from build123d import *

# Parameters (mm, degrees)
SKETCH_W      = 85
SKETCH_H      = 56
SKETCH_R      = 1.35
PAD_DEPTH     = 4
SKETCH001_W   = 50
SKETCH001_H   = 5
PAD001_DEPTH  = 8.5
SKETCH002_W   = 50
SKETCH002_H   = 5
SKETCH002_W_2 = 48
SKETCH002_H_2 = 3
POCKET_DEPTH  = 6
SKETCH003_W   = 17.5
SKETCH003_H   = 12
PAD002_DEPTH  = 16
SKETCH004_W   = 21.1
SKETCH004_H   = 16
PAD003_DEPTH  = 13.5
SKETCH005_W   = 9.2
SKETCH005_H   = 10.5
PAD004_DEPTH  = 3.2
SKETCH006_W   = 7
SKETCH006_H   = 8
PAD005_DEPTH  = 3
SKETCH007_W   = 7
SKETCH007_H   = 12
PAD006_DEPTH  = 6


with BuildPart() as part:
    # Sketch → Pad (new body)
    with BuildSketch(Plane.XY):
        Rectangle(SKETCH_W, SKETCH_H)
        with Locations((-39, 24.5)):
            Circle(SKETCH_R, mode=Mode.SUBTRACT)
        with Locations((19, 24.5)):
            Circle(SKETCH_R, mode=Mode.SUBTRACT)
        with Locations((-39, -24.5)):
            Circle(SKETCH_R, mode=Mode.SUBTRACT)
        with Locations((19, -24.5)):
            Circle(SKETCH_R, mode=Mode.SUBTRACT)
    extrude(amount=-PAD_DEPTH)

    # Sketch001 (on Face9 of Pad) → Pad001 (join)
    with BuildSketch(Plane.XY):
        with Locations((-10, 24.5)):
            Rectangle(SKETCH001_W, SKETCH001_H)
    extrude(amount=PAD001_DEPTH)

    # Sketch002 (on Face15 of Pad001) → Pocket (cut)
    with BuildSketch(Plane.XY.offset(8.5)):
        with Locations((-10, 24.5)):
            Rectangle(SKETCH002_W, SKETCH002_H)
        with Locations((-10, 24.5)):
            Rectangle(SKETCH002_W_2, SKETCH002_H_2, mode=Mode.SUBTRACT)
    extrude(amount=-POCKET_DEPTH, mode=Mode.SUBTRACT)

    # Sketch003 (on Face4 of Pocket) → Pad002 (join)
    with BuildSketch(Plane.XY):
        with Locations((37.25, 19)):
            Rectangle(SKETCH003_W, SKETCH003_H)
        with Locations((37.25, 1)):
            Rectangle(SKETCH003_W, SKETCH003_H)
    extrude(amount=PAD002_DEPTH)

    # Sketch004 (on Face4 of Pad002) → Pad003 (join)
    with BuildSketch(Plane.XY):
        with Locations((35.45, -17.75)):
            Rectangle(SKETCH004_W, SKETCH004_H)
    extrude(amount=PAD003_DEPTH)

    # Sketch005 (on Face4 of Pad003) → Pad004 (join)
    with BuildSketch(Plane.XY):
        with Locations((-31.3, -23.75)):
            Rectangle(SKETCH005_W, SKETCH005_H)
    extrude(amount=PAD004_DEPTH)

    # Sketch006 (on Face4 of Pad004) → Pad005 (join)
    with BuildSketch(Plane.XY):
        with Locations((-16.5, -25)):
            Rectangle(SKETCH006_W, SKETCH006_H)
        with Locations((-3, -25)):
            Rectangle(SKETCH006_W, SKETCH006_H)
    extrude(amount=PAD005_DEPTH)

    # Sketch007 (on Face4 of Pad005) → Pad006 (join)
    with BuildSketch(Plane.XY):
        with Locations((11.5, -23)):
            Rectangle(SKETCH007_W, SKETCH007_H)
    extrude(amount=PAD006_DEPTH)


solid = part.part
The model under review builds one solid part; all positions refer to its coordinate system, in mm. A direction names the side the tool comes from. Give positions to 0.01 mm unless a question says otherwise; leave off trailing zeros. Loops run counter-clockwise (first coordinate to the right, second up) from the corner with the lowest first, then second, coordinate; pieces in that order, holes last. Notation, with made-up numbers: (-5.75, -4.75) -> (20.25, -4.75) arc R27 ccw to (20.25, 14.25) -> close; hole circle Ø9 at (-13, -19). An arc over 180 degrees is marked (long way). Put each result on its own line as item: value. Start each with the question number.
1. Wall thickness on probe 1 along Y at (x, z) = (-39, -2.05); probe 2 along Y at (x, z) = (34, 3.25); probe 3 along Y at (x, z) = (8.5, 1.5): over which ranges is each line inside the solid? List them lowest first.
2. Clearance check with flat-ended pins moving along their axes: P1, Ø4.5, axis at x = 1.5, z = -2.5, coming from the -Y side; P2, Ø10, axis at y = -18.5, z = 7, coming from the -X side; P3, Ø1, axis at x = 44.5, y = 21.5, coming from the -Z side. State where each tip first meets the part, or that it passes through.
3. We need section A-A on x = 19. State the section outline as (y, z) points, then the cut area to 3 significant figures.
4. Mouldability with a two-part tool opening along X and no side actions: class faces 4 (the face through (-34, 24, 6)), 5 (the face through (0.5, -25, 1)), 6 (the face through (44, 1, 0)), 7 (the face through (46, 1, 8)) as released by +X, released by -X, zero draft, split by the parting line, or undercut.
5. For faces 1 (the face through (-31, -24, 3.2)), 2 (the face through (42.5, 0, -2)), 3 (the face through (37, 13, 8)), list the 3-axis set-ups (+Z, -Z, +X, -X, +Y, -Y) from which the entire face can be reached by the end or side of a thin tool; tool diameter is ignored.
6. We need section D-D on x = 34.5. State the section outline as (y, z) points, then the cut area to 3 significant figures.
7. We need section B-B on z = 10.25. State the section outline as (x, y) points, then the cut area to 3 significant figures.
8. We need section C-C on y = -24.5. State how many separate pieces and enclosed holes the cut face has, then the cut area to 3 significant figures.
Determined:
1. probe 1: -28 to -25.85, -23.15 to 23.15, 25.85 to 28
1. probe 2: -25.75 to -9.75, -5 to 7, 13 to 25
1. probe 3: -29 to -17, 22 to 27
2. P1: y = -28
2. P2: x = -35.9
2. P3: z = 0
3. outline: (-28, -4) -> (-25.85, -4) -> (-25.85, 0) -> (-28, 0) -> close; (-23.15, -4) -> (23.15, -4) -> (23.15, 0) -> (-23.15, 0) -> close; (25.85, -4) -> (28, -4) -> (28, 0) -> (25.85, 0) -> close
3. area: 202 mm^2
4. face 4: released by -X
4. face 5: undercut
4. face 6: zero draft
4. face 7: released by +X
5. face 1: +Z, -X, -Y
5. face 2: -Z, +X, +Y, -Y
5. face 3: +Z, +X, -X
6. outline: (-28, -4) -> (28, -4) -> (28, 0) -> (25, 0) -> (25, 16) -> (13, 16) -> (13, 0) -> (7, 0) -> (7, 16) -> (-5, 16) -> (-5, 0) -> (-9.75, 0) -> (-9.75, 13.5) -> (-25.75, 13.5) -> (-25.75, 0) -> (-28, 0) -> close
6. area: 824 mm^2
7. outline: (24.9, -25.75) -> (46, -25.75) -> (46, -9.75) -> (24.9, -9.75) -> close; (28.5, -5) -> (46, -5) -> (46, 7) -> (28.5, 7) -> close; (28.5, 13) -> (46, 13) -> (46, 25) -> (28.5, 25) -> close
7. area: 758 mm^2
8. separate pieces: 3
8. enclosed holes: 0
8. area: 717 mm^2
